The drawing under review shows one solid part. Ordinate dimensions are in mm from its lowest x, y, z. A direction names the side the tool comes from. Give positions to 0.01 mm unless a question says otherwise; leave off trailing zeros. Loops run counter-clockwise (first coordinate to the right, second up) from the corner with the lowest first, then second, coordinate; pieces in that order, holes last. Notation, with made-up numbers: (-38, 63) - (-32, 63) arc R17 ccw to (-32, 92) - close; hole circle Ø1 at (87, 5). An arc over 180 degrees is marked (long way). Answer as CSV lines item,"result".
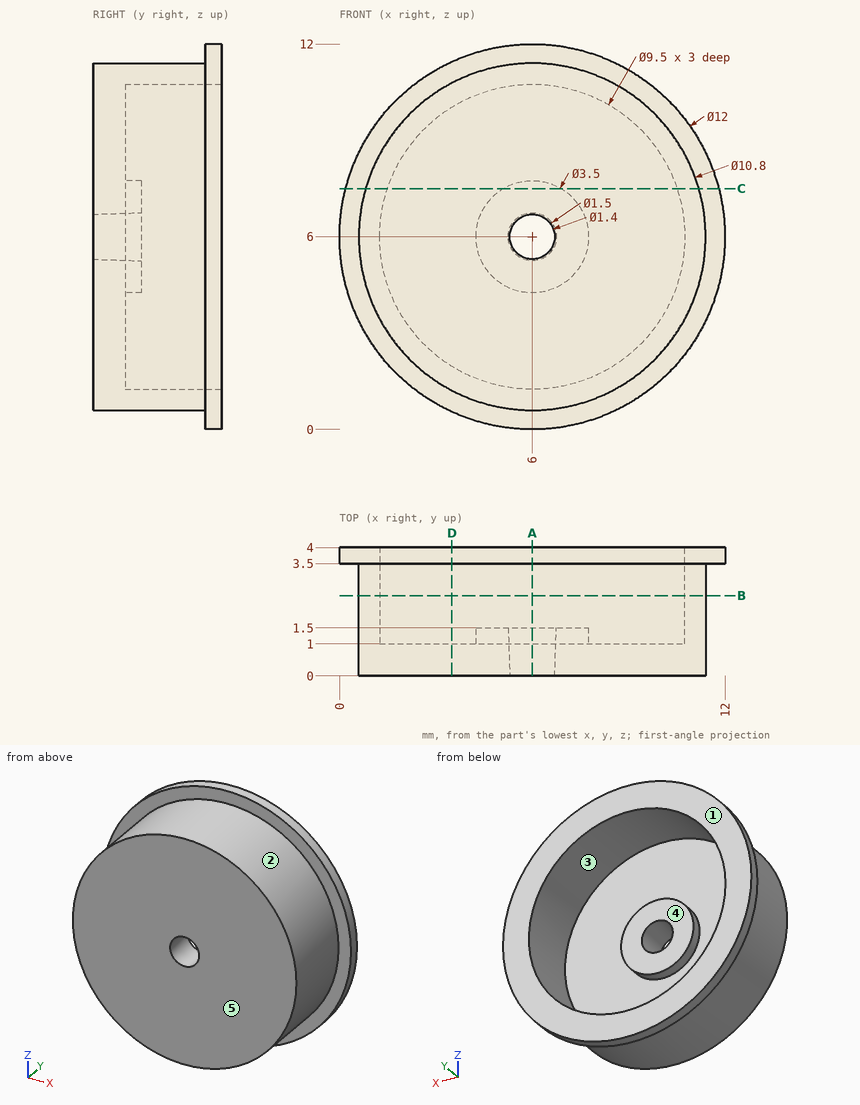
1) Machinability: for the marked faces 4 and 5, which of the approach directions +Z, -Z, +X, -X, +Y, -Y give a long, thin tool a straight path to every point of the face, cutting with its end or side? Answer none if there is none.
From the geometry:
face 4,"+Y"
face 5,"+Z, -Z, +X, -X, -Y"
2) Draft analysis for pull direction Z (two halves, no side actions). For the marked faces 1, 2 and 3, state which applies: pulls with the +Z half, pulls with the -Z half, needs draft (parallel to the pull), parting line crosses it, or undercut.
From the geometry:
face 1,"needs draft"
face 2,"parting line crosses it"
face 3,"undercut"
3) Consider section D-D on x = 3.5. Write out the cut boundary in (y, z), and give its area (3 significant figures).
From the geometry:
outline,"(0, 1.21) - (3.5, 1.21) - (3.5, 0.55) - (4, 0.55) - (4, 1.96) - (1, 1.96) - (1, 10.04) - (4, 10.04) - (4, 11.45) - (3.5, 11.45) - (3.5, 10.79) - (0, 10.79) - close"
area,"14.7 mm^2"
4) Consider section C-C on z = 7.5. Write out the cut boundary in (x, y), and give its area (3 significant figures).
From the geometry:
outline,"(0.19, 3.5) - (0.81, 3.5) - (0.81, 0) - (11.19, 0) - (11.19, 3.5) - (11.81, 3.5) - (11.81, 4) - (10.51, 4) - (10.51, 1) - (6.9, 1) - (6.9, 1.5) - (5.1, 1.5) - (5.1, 1) - (1.49, 1) - (1.49, 4) - (0.19, 4) - close"
area,"16.0 mm^2"
5) Wall thickness on line 1 (Z direction, x = 6, y = 1.85); line 2 (Z direction, x = 7, y = 1.45); line 3 (Y direction, x = 10, z = 6.25): over which ranges is each line inside the solid? List them lowest first. Write a range as from..to.
From the geometry:
line 1,"z = 0.6..1.25, 10.75..11.4"
line 2,"z = 0.69..1.36, 4.56..7.44, 10.64..11.31"
line 3,"y = 0..1"
6) Consider section A-A on x = 6. Write out the cut boundary in (y, z), and give its area (3 significant figures).
From the geometry:
outline,"(0, 0.6) - (3.5, 0.6) - (3.5, 0) - (4, 0) - (4, 1.25) - (1, 1.25) - (1, 4.25) - (1.5, 4.25) - (1.5, 5.25) - (0, 5.3) - close; (0, 6.7) - (1.5, 6.75) - (1.5, 7.75) - (1, 7.75) - (1, 10.75) - (4, 10.75) - (4, 12) - (3.5, 12) - (3.5, 11.4) - (0, 11.4) - close"
area,"14.9 mm^2"
7) Insertion check: P1, Ø1, axis at x = 5.5, z = 5.5, coming from the +Y side; P2, Ø2, axis at x = 7.5, y = 3, coming from the +Z side; P3, Ø1.5, axis at y = 2.5, z = 8.5, coming from the -X side. Each pin has a flat end and moves straight along its axis. Give the tip position at first contact, or say it passes through.
From the geometry:
P1,"stops at y = 1.5"
P2,"stops at z = 11.97"
P3,"stops at x = 0.89"
8) Consider section B-B on y = 2.5. Write out the cut boundary in (x, z), and give its area (3 significant figures).
From the geometry:
outline,"circle Ø10.8 at (6, 6); hole circle Ø9.5 at (6, 6)"
area,"20.7 mm^2"
